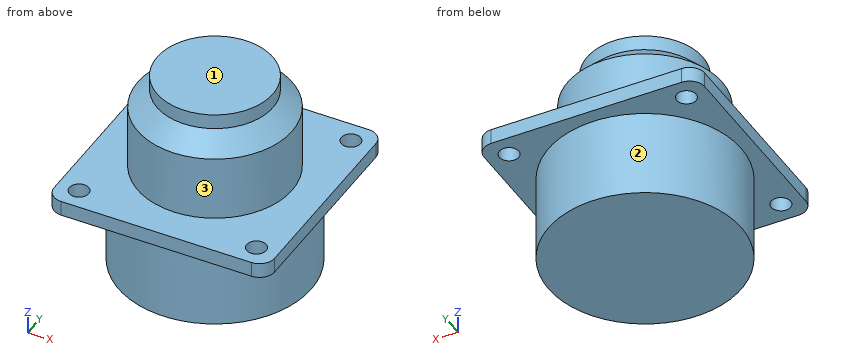
from build123d import *

# Parameters (mm, degrees)
SKETCH2_OUTSIDE_W  = 68.636
SKETCH2_OUTSIDE_H  = 68.636
CUT_EXTRUDE2_DEPTH = 41.588659571
SKETCH4_R          = 1.6002
CUT_EXTRUDE4_DEPTH = 32.872258651


with BuildPart() as part:
    # Sketch1 → Revolve1 (revolve)
    with BuildSketch(Plane(origin=(0, 0, 0), x_dir=(0, 0, -1), z_dir=(1, 0, 0)), mode=Mode.PRIVATE) as revolve1_sk:
        Polygon((-2.4892, 25.4), (0, 25.4), (0, 15.8496), (14.4018, 15.8496), (14.4018, 0), (-18.8976, 0), (-18.8976, 9.525), (-16.4084, 9.525), (-13.2334, 12.7), (-2.4892, 12.7), align=None)
    revolve(revolve1_sk.sketch.rotate(Axis((0, 0, 0), (0, 0, 1)), 90), axis=Axis((0, 0, 0), (0, 0, 1)))

    # Sketch2 outside → Cut-Extrude2 (cut, through all)
    with BuildSketch(Plane.XY):
        Rectangle(SKETCH2_OUTSIDE_W, SKETCH2_OUTSIDE_H)
        with BuildLine():
            Line((-15.6591, 18.1483), (15.6591, 18.1483))
            ThreePointArc((15.6591, 18.1483), (17.4192302, 17.4192302), (18.1483, 15.6591))
            Line((18.1483, 15.6591), (18.1483, -15.6591))
            ThreePointArc((18.1483, -15.6591), (17.4192302, -17.4192302), (15.6591, -18.1483))
            Line((15.6591, -18.1483), (-15.6591, -18.1483))
            ThreePointArc((-15.6591, -18.1483), (-17.4192302, -17.4192302), (-18.1483, -15.6591))
            Line((-18.1483, -15.6591), (-18.1483, 15.6591))
            ThreePointArc((-18.1483, 15.6591), (-17.4192302, 17.4192302), (-15.6591, 18.1483))
        make_face(mode=Mode.SUBTRACT)
    extrude(amount=CUT_EXTRUDE2_DEPTH, mode=Mode.SUBTRACT)

    # Sketch4 → Cut-Extrude4 (cut, through all)
    with BuildSketch(Plane.XY):
        with Locations((-14.605, 14.605)):
            Circle(SKETCH4_R)
        with Locations(Location((14.605, 14.605, 0), (0, 0, 180))):
            Circle(SKETCH4_R)
        with Locations(Location((-14.605, -14.605, 0), (0, 0, 180))):
            Circle(SKETCH4_R)
        with Locations((14.605, -14.605)):
            Circle(SKETCH4_R)
    extrude(amount=CUT_EXTRUDE4_DEPTH, mode=Mode.SUBTRACT)


solid = part.part
For this review, take the finished solid that the model builds, in its own axes (mm). Face numbers are marked on the shaded views. A direction names the side the tool comes from. Round coordinates to 2 decimals unless told otherwise and drop trailing zeros. Order: outer loops, then holes, each group sorted by start corner. A loop starts at its lowest first (then second) coordinate and runs counter-clockwise, first axis right, second up. Notation, with made-up numbers: M 69,75.5 L 99,75.5 A21 ccw 99,106.5 Z; hole C -21.5,-23.5 d6. An arc over 180 degrees is marked long. Use a Markdown table: item, result. Add a question column.
Item 1: Insertion check: pin 1 (4 mm diameter, centred on x = 14.605, y = 14.605, fed in from -Z); pin 2 (4 mm diameter, centred on x = 14.605, y = -14.605, fed in from +Z); pin 3 (4 mm diameter, centred on y = 14, z = -11, fed in from +X). Each pin has a flat end and moves straight along its axis. Give the tip position at first contact, or say it passes through.
Item 2: Add section B-B, the plane y = 0. Give the boundary of the cut face in (x, z) (3 decimals), then the cut area to 3 significant figures.
Item 3: Add section D-D, the plane z = 12. Give the boundary of the cut face in (x, y).
Item 4: Tool access review of the marked faces 1, 2 and 3: name each direction out of +Z, -Z, +X, -X, +Y, -Y from which nothing blocks a thin tool from reaching the whole face with its end or side.
Item 5: To check wall thickness, follow line 1 along Z through (x, y) = (13, -4.5); line 2 along Y through (x, z) = (0.5, -3.5); line 3 along Z through (x, y) = (14, 12). State the ranges of each line that lie inside material, in increasing order.
Item 6: Add section A-A, the plane x = -14.5. Give the boundary of the cut face in (y, z), then the cut area to 3 significant figures.
Geometry results:
| question | item | result |
|---|---|---|
| 1 | pin 1 | stops at z = 0 |
| 1 | pin 2 | stops at z = 2.49 |
| 1 | pin 3 | stops at x = 10.35 |
| 2 | outline | M -18.148,0 L -15.85,0 L -15.85,-14.402 L 15.85,-14.402 L 15.85,0 L 18.148,0 L 18.148,2.489 L 12.7,2.489 L 12.7,13.233 L 9.525,16.408 L 9.525,18.898 L -9.525,18.898 L -9.525,16.408 L -12.7,13.233 L -12.7,2.489 L -18.148,2.489 Z |
| 2 | area | 938 mm² |
| 3 | outline | C 0,0 d25.4 |
| 4 | face 1 | +Z, +X, -X, +Y, -Y |
| 4 | face 2 | -Z |
| 4 | face 3 | +Z |
| 5 | line 1 | z = -14.4 to 2.49 |
| 5 | line 2 | y = -15.84 to 15.84 |
| 5 | line 3 | z = 0 to 2.49 |
| 6 | outline | M -18.15,0 L -16.2,0 L -16.2,2.49 L -18.15,2.49 Z; M -13.01,0 L -6.4,0 L -6.4,-14.4 L 6.4,-14.4 L 6.4,0 L 13.01,0 L 13.01,2.49 L -13.01,2.49 Z; M 16.2,0 L 18.15,0 L 18.15,2.49 L 16.2,2.49 Z |
| 6 | area | 259 mm² |
